CAD build for the part. Positions are in the model's coordinates, mm. Round coordinates to 2 decimals unless told otherwise and drop trailing zeros. Write each loop counter-clockwise with the first axis right and the second up, starting at its lowest first coordinate (ties: lowest second). Pieces come first, ordered by that corner, then holes. Notation, with made-up numbers: (-6, 76) -> (13, 76) arc R21 ccw to (13, 115) -> close; hole circle Ø8 at (0.25, 28). An arc over 180 degrees is marked (long way). Answer in a Markdown table with one row per item. Add a question column.
```python
from build123d import *

# Parameters (mm, degrees)
F0_W     = 42.8752
F0_H     = 42.8752
F0_R     = 10.7188
F1_DEPTH = 21.4376


with BuildPart() as f1:
    # F0 (on Front) → F1 (new body)
    with BuildSketch(Plane.XZ):
        with Locations((21.4376, 0)):
            Rectangle(F0_W, F0_H)
        with Locations((21.4376, 0)):
            Circle(F0_R, mode=Mode.SUBTRACT)
        with Locations((-21.4376, 0)):
            Rectangle(F0_W, F0_H)
        with Locations((-21.4376, 0)):
            Circle(F0_R, mode=Mode.SUBTRACT)
    extrude(amount=F1_DEPTH)


solid = f1.part
```
Item 1: Saw through at B-B on x = 21.5. Give the cut face in (y, z).
Item 2: Saw through at A-A on z = 0. Give the cut face in (x, y).
Item 3: Two-plate mould, pull along X, no slides. Class faces 1 (the cylindrical face through (10.73, -10.57, 0.47)), 2 (the flat face through (-42.875, -11, 0)), 3 (the flat face through (-1, -11, -21.438)): +X half, -X half, draft (parallel to the pull), parting line (faces both ways), or undercut.
Item 4: Pin check, flat tip, straight feed: pin 1 (5 mm diameter, centred on x = -8.5, z = 7.5, fed in from +Y). Stop position of the tip, or through.
Item 5: Saw through at C-C on y = -19. Give the cut face in (x, z), then the cut area to 3 significant figures.
Item 6: Drill centre lines: probe 1 along Z at (x, y) = (22, -16.75); probe 2 along X at (y, z) = (-12.75, 3.5); probe 3 along X at (y, z) = (-6.5, 6.5). Where is each one in solid material? Low to high.
Item 7: Saw through at D-D on z = 5.5. Give the cut face in (x, y).
Recorded:
| question | item | result |
|---|---|---|
| 1 | outline | (-21.44, -21.44) -> (0, -21.44) -> (0, -10.72) -> (-21.44, -10.72) -> close; (-21.44, 10.72) -> (0, 10.72) -> (0, 21.44) -> (-21.44, 21.44) -> close |
| 2 | outline | (-42.88, -21.44) -> (-32.16, -21.44) -> (-32.16, 0) -> (-42.88, 0) -> close; (-10.72, -21.44) -> (10.72, -21.44) -> (10.72, 0) -> (-10.72, 0) -> close; (32.16, -21.44) -> (42.88, -21.44) -> (42.88, 0) -> (32.16, 0) -> close |
| 3 | face 1 | undercut |
| 3 | face 2 | -X half |
| 3 | face 3 | draft |
| 4 | pin 1 | y = 0 |
| 5 | outline | (-42.88, -21.44) -> (42.88, -21.44) -> (42.88, 21.44) -> (-42.88, 21.44) -> close; hole circle Ø21.44 at (-21.44, 0); hole circle Ø21.44 at (21.44, 0) |
| 5 | area | 2,950 mm2 |
| 6 | probe 1 | -21.44 to -10.7, 10.7 to 21.44 |
| 6 | probe 2 | -42.88 to -31.57, -11.31 to 11.31, 31.57 to 42.88 |
| 6 | probe 3 | -42.88 to -29.96, -12.91 to 12.91, 29.96 to 42.88 |
| 7 | outline | (-42.88, -21.44) -> (-30.64, -21.44) -> (-30.64, 0) -> (-42.88, 0) -> close; (-12.24, -21.44) -> (12.24, -21.44) -> (12.24, 0) -> (-12.24, 0) -> close; (30.64, -21.44) -> (42.88, -21.44) -> (42.88, 0) -> (30.64, 0) -> close |
